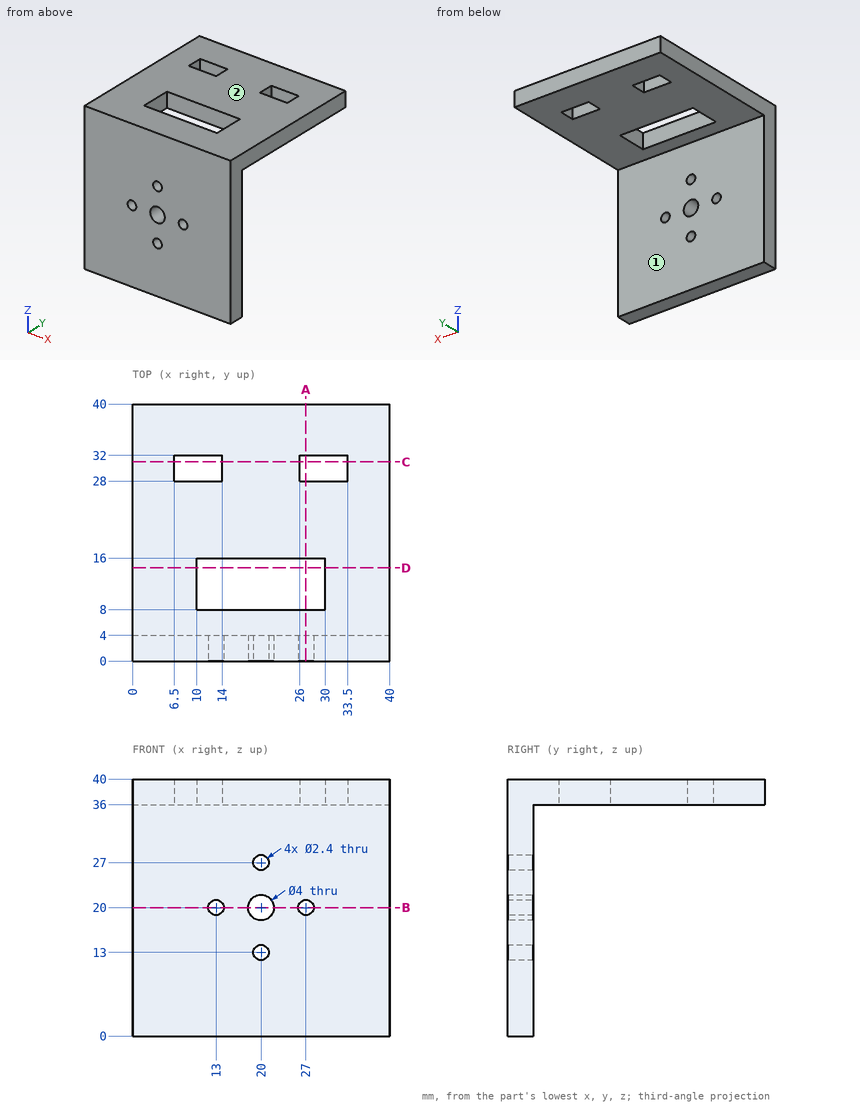
Part print with two shaded views. Sizes in mm from the minimum x, y, z corner. A direction names the side the tool comes from. Coordinates: 2 decimals unless noted, no trailing zeros. Write each loop counter-clockwise with the first axis right and the second up, starting at its lowest first coordinate (ties: lowest second). Pieces come first, ordered by that corner, then holes.
(1) Pin check, flat tips, straight feed: pin 1 Ø5 at (x, y) = (20, 15.5) entering from -Z; pin 2 Ø2 at (x, z) = (14, 22) entering from -Y; pin 3 Ø3 at (x, z) = (27, 20) entering from +Y. Stop position of each tip, or through.
(2) Cut at C-C on y = 31. List the corners of the cut face in (x, z), and give its area (3 significant figures).
(3) 3-axis set-ups, long thin cutter, end or side, ignore diameter. For the marked faces 1 and 2: which of +Z, -Z, +X, -X, +Y, -Y reach the whole face in a straight line?
(4) Cut at A-A on x = 27. List the corners of the cut face in (y, z), and give its area (3 significant figures).
(5) Cut at B-B on z = 20. List the corners of the cut face in (x, y), and give its area (3 significant figures).
(6) Drill centre lines: line 1 (X direction, y = 1.95, z = 20); line 2 (Z direction, x = 20.5, y = 2); line 3 (Y direction, x = 4.5, z = 32). Where is each one in solid material? Low to high.
(7) Cut at D-D on y = 14.5. List the corners of the cut face in (x, z), and give its area (3 significant figures).
Working result:
1. pin 1: stops at z = 36
1. pin 2: stops at y = 0
1. pin 3: stops at y = 4
2. outline: (0, 36) - (6.5, 36) - (6.5, 40) - (0, 40) - close; (14, 36) - (26, 36) - (26, 40) - (14, 40) - close; (33.5, 36) - (40, 36) - (40, 40) - (33.5, 40) - close
2. area: 100 mm2
3. face 1: -Z, +X, -X, +Y
3. face 2: +Z, +X, -X, +Y, -Y
4. outline: (0, 0) - (4, 0) - (4, 18.8) - (0, 18.8) - close; (0, 21.2) - (4, 21.2) - (4, 36) - (8, 36) - (8, 40) - (0, 40) - close; (16, 36) - (28, 36) - (28, 40) - (16, 40) - close; (32, 36) - (40, 36) - (40, 40) - (32, 40) - close
4. area: 246 mm2
5. outline: (0, 0) - (11.8, 0) - (11.8, 4) - (0, 4) - close; (14.2, 0) - (18, 0) - (18, 4) - (14.2, 4) - close; (22, 0) - (25.8, 0) - (25.8, 4) - (22, 4) - close; (28.2, 0) - (40, 0) - (40, 4) - (28.2, 4) - close
5. area: 125 mm2
6. line 1: x = 0 to 11.8, 14.2 to 18, 22 to 25.8, 28.2 to 40
6. line 2: z = 0 to 11.91, 14.09 to 18.06, 21.94 to 25.91, 28.09 to 40
6. line 3: y = 0 to 4
7. outline: (0, 36) - (10, 36) - (10, 40) - (0, 40) - close; (30, 36) - (40, 36) - (40, 40) - (30, 40) - close
7. area: 80.0 mm2
